Input: part model. Units: mm. Frame: model coordinates. A direction names the side the tool comes from. Give positions to 0.01 mm unless a question says otherwise; leave off trailing zeros. Loops run counter-clockwise (first coordinate to the right, second up) from the corner with the lowest first, then second, coordinate; pieces in that order, holes last. Notation, with made-up numbers: (14.25, 35.5) - (44.25, 35.5) arc R20 cw to (44.25, 65.5) - close; hole circle Ø2 at (8, -9.5). An arc over 180 degrees is marked (long way). Answer as a JSON object with one key per item and string values. Group by question number.
(1) Section query C-C (y = 42). Return loops of the section in (x, z), plus the area to 3 significant figures.
(2) Section query A-A (z = 0). Return loops of the section in (x, y), plus the area to 3 significant figures.
(3) Pin query (flat end, axial travel): P1, Ø14, axis at x = 0, y = 30, coming from the -Z side; P2, Ø4.5, axis at x = -3.5, z = -18.5, coming from the +Y side; P3, Ø6, axis at x = 13, z = -3, coming from the -Y side. Return the tip coordinate at first contact, or that it passes through.
(4) Mould query, pull axis X, two halves, no side actions, for faces 4 (the flat face through (0, 25, 20)), 5 (the cylindrical face through (-0.191, 25.654, 17.972)), 6 (the cylindrical face through (0, 50, 18)). Classes: +X half, -X half, draft (parallel to the pull), parting line (faces both ways), or undercut.
(5) Material intervals for L1, parallel to Z at x = -5.5, y = 40.5; L2, parallel to X at y = 30, z = -13.5; L3, parallel to Y at x = 17.5, z = 2, sorted ascending.
(6) Section query D-D (y = 32). Return loops of the section in (x, z), plus the area to 3 significant figures.
(7) Access query for faces 1 (the flat face through (0, 22, -16)), 2 (the flat face through (-20, 3.8, 0.1)), 3 (the flat face through (0, 22, -12)). Directions: +Z, -Z, +X, -X, +Y, -Y. A direction counts if a zero-diameter tool reaches every point of the face in a straight line with its end or side. Return the directions, or none.
(8) Section query B-B (x = 0). Return loops of the section in (y, z), plus the area to 3 significant figures.
```python
from build123d import *

# Parameters (mm, degrees)
SKETCH1_W               = 40
SKETCH1_H               = 30
BOSS_EXTRUDE1_DEPTH     = 20
CUT_EXTRUDE1_DEPTH      = 58.445626465
CUT_EXTRUDE1_DEPTH_BACK = 58.445626465
SKETCH2_W               = 28
SKETCH2_H               = 46
SKETCH2_W_2             = 4
CUT_EXTRUDE2_DEPTH      = 68.082039325
CUT_EXTRUDE2_DEPTH_BACK = 68.082039325
SKETCH3_R               = 4.35
SKETCH4_R               = 4.35
CUT_EXTRUDE3_DEPTH      = 58.445626465


with BuildPart() as part:
    # Sketch1 → Boss-Extrude1 (new, symmetric)
    with BuildSketch(Plane.XY):
        with BuildLine():
            ThreePointArc((-20, 30), (0, 50), (20, 30))
            Line((20, 30), (-20, 30))
        make_face()
        with Locations((0, 15)):
            Rectangle(SKETCH1_W, SKETCH1_H)
    extrude(amount=BOSS_EXTRUDE1_DEPTH, both=True)

    # Sketch2 → Cut-Extrude1 (cut, two sides: drawn at the far end of the back side and taken through both)
    with BuildSketch(Plane(origin=(0, 0, 0), x_dir=(0, 0, -1), z_dir=(1, 0, 0)).offset(-CUT_EXTRUDE1_DEPTH_BACK)):
        with Locations((-2, 27)):
            Rectangle(SKETCH2_W, SKETCH2_H)
        with Locations((18, 27)):
            Rectangle(SKETCH2_W_2, SKETCH2_H)
    extrude(amount=CUT_EXTRUDE1_DEPTH + CUT_EXTRUDE1_DEPTH_BACK, mode=Mode.SUBTRACT)

    # Sketch3 → Cut-Extrude2 (cut, two sides: drawn at the far end of the back side and taken through both)
    with BuildSketch(Plane.XY.offset(20).offset(-CUT_EXTRUDE2_DEPTH_BACK)):
        with Locations(Location((0, 30, 0), (0, 0, 90))):
            Circle(SKETCH3_R)
    extrude(amount=CUT_EXTRUDE2_DEPTH + CUT_EXTRUDE2_DEPTH_BACK, mode=Mode.SUBTRACT)

    # Sketch4 → Cut-Extrude3 (cut, through all)
    with BuildSketch(Plane.XZ):
        with Locations(Location((0, 0, 0), (0, 0, 270))):
            Circle(SKETCH4_R)
    extrude(amount=-CUT_EXTRUDE3_DEPTH, mode=Mode.SUBTRACT)


solid = part.part
```
Recorded:
{
 "1": {"outline": "(-16, -16) - (16, -16) - (16, -12) - (-16, -12) - close; (-16, 16) - (16, 16) - (16, 20) - (-16, 20) - close", "area": "256 mm^2"},
 "2": {"outline": "(-20, 0) - (-4.35, 0) - (-4.35, 4) - (-20, 4) - close; (4.35, 0) - (20, 0) - (20, 4) - (4.35, 4) - close", "area": "125 mm^2"},
 "3": {"P1": "stops at z = -16", "P2": "stops at y = 4", "P3": "stops at y = 0"},
 "4": {"face 4": "draft", "face 5": "undercut", "face 6": "parting line"},
 "5": {"L1": "z = -16 to -12, 16 to 20", "L2": "x = -20 to -4.35, 4.35 to 20", "L3": "y = 0 to 4"},
 "6": {"outline": "(-19.9, -16) - (-3.86, -16) - (-3.86, -12) - (-19.9, -12) - close; (-19.9, 16) - (-3.86, 16) - (-3.86, 20) - (-19.9, 20) - close; (3.86, -16) - (19.9, -16) - (19.9, -12) - (3.86, -12) - close; (3.86, 16) - (19.9, 16) - (19.9, 20) - (3.86, 20) - close", "area": "257 mm^2"},
 "7": {"face 1": "-Z, +X, -X, +Y", "face 2": "+Z, -Z, -X, +Y, -Y", "face 3": "+X, -X, +Y"},
 "8": {"outline": "(0, -20) - (4, -20) - (4, -16) - (25.65, -16) - (25.65, -12) - (4, -12) - (4, -4.35) - (0, -4.35) - close; (0, 4.35) - (4, 4.35) - (4, 16) - (25.65, 16) - (25.65, 20) - (0, 20) - close; (34.35, -16) - (50, -16) - (50, -12) - (34.35, -12) - close; (34.35, 16) - (50, 16) - (50, 20) - (34.35, 20) - close", "area": "424 mm^2"}
}
